Verification items for the finished model (mm, model axes). Round coordinates to 2 decimals unless told otherwise and drop trailing zeros. Write each loop counter-clockwise with the first axis right and the second up, starting at its lowest first coordinate (ties: lowest second). Pieces come first, ordered by that corner, then holes. Notation, with made-up numbers: M 3.25,5 L 11.25,5 A29 cw 11.25,28 Z; hole C -16.5,73 d10. An arc over 180 degrees is marked long. One line per item, written item: value. Start each with the question number.
Item 1: Section check A-A, the plane z = 0.95. State how many separate pieces and enclosed holes the cut face has, then the cut area to 3 significant figures.
Item 2: Thickness scan on probe 1 along X at (y, z) = (254, 1.2); probe 2 along Y at (x, z) = (228.6, 2.45); probe 3 along X at (y, z) = (368.3, 0.7). Record the ranges inside material, lowest first. Write a range as from..to.
Item 3: Gauge pin test, flat ends, axial feed: pin 1 (11.5 mm diameter, centred on x = 571.5, y = 25.4, fed in from +Z) (3 decimals); pin 2 (1 mm diameter, centred on x = 46.5, z = 1, fed in from +Y); pin 3 (6.5 mm diameter, centred on x = 774.7, y = 254, fed in from +Z). Record the tip position at first contact, or that the pin passes through.
Item 4: Section check B-B, the plane x = 585.5. Record the cut outline in (y, z) (3 decimals), then the cut area to 3 significant figures.
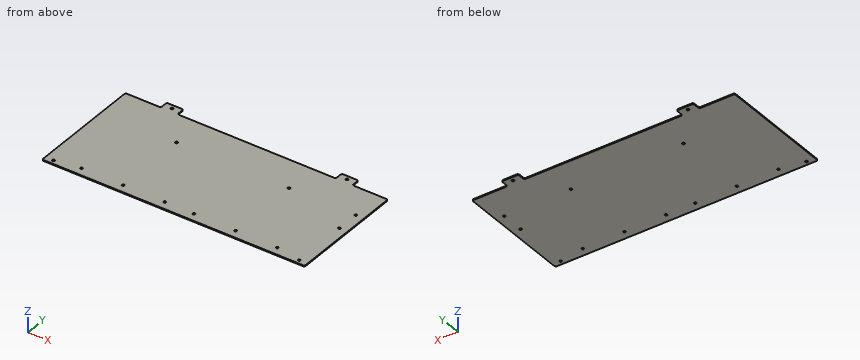
from build123d import *

# Parameters (mm, degrees)
F0_W     = 107.95
F0_H     = 355.6
F0_W_2   = 50.8
F0_H_2   = 25.4
F1_DEPTH = 3.175
F2_D     = 7.1374
F3_R     = 5.08
F5_D     = 7.1374


# Not quite as in the source:
# - a feature names something its author has since deleted; it is built from what else it names


with BuildPart() as f1:
    # F0 (on Top) → F1 (new body)
    with BuildSketch(Plane.XY):
        with Locations((53.975, 177.8)):
            Rectangle(F0_W, F0_H)
        Polygon((107.95, 355.6), (107.95, 0), (400.05, 0), (400.05, 355.6), (158.75, 355.6), align=None)
        with Locations((133.35, 368.3)):
            Rectangle(F0_W_2, F0_H_2)
        Polygon((400.05, 355.6), (400.05, 0), (692.15, 0), (692.15, 355.6), (641.35, 355.6), align=None)
        with Locations((746.125, 177.8)):
            Rectangle(F0_W, F0_H)
        with Locations((666.75, 368.3)):
            Rectangle(F0_W_2, F0_H_2)
    extrude(amount=F1_DEPTH)

    # F2 (through all)
    with Locations(Plane(origin=(0, 0, 0), x_dir=(1, 0, 0), z_dir=(0, 0, -1))):
        with Locations((133.35, -368.3), (666.75, -368.3), (25.4, -12.7), (774.7, -12.7)):
            Hole(F2_D / 2)

    # F3
    f3_edges = [f1.edges().sort_by_distance(p)[0] for p in [
        (0, 355.6, 1.5875),
        (107.95, 355.6, 1.5875),
        (107.95, 381, 1.5875),
        (158.75, 381, 1.5875),
        (158.75, 355.6, 1.5875),
        (692.15, 355.6, 1.5875),
        (692.15, 381, 1.5875),
        (641.35, 381, 1.5875),
        (641.35, 355.6, 1.5875),
        (800.1, 355.6, 1.5875),
        (800.1, 0, 1.5875),
        (0, 0, 1.5875),
    ]]
    fillet(f3_edges, radius=F3_R)

    # F5 (through all)
    with Locations(Plane.XY.offset(3.175)):
        with Locations((571.5, 254), (774.7, 254), (444.5, 25.4), (571.5, 25.4), (698.5, 25.4), (774.7, 184.15), (101.6, 25.4), (228.6, 25.4), (355.6, 25.4), (228.6, 254)):
            Hole(F5_D / 2)


solid = f1.part
Response values:
1. separate pieces: 1
1. enclosed holes: 14
1. area: 287,000 mm2
2. probe 1: x = 0..225.03, 232.17..567.93, 575.07..771.13, 778.27..800.1
2. probe 2: y = 0..21.83, 28.97..250.43, 257.57..355.6
2. probe 3: x = 107.95..129.78, 136.92..158.75, 641.35..663.18, 670.32..692.15
3. pin 1: stops at z = 3.175
3. pin 2: stops at y = 355.6
3. pin 3: passes through
4. outline: M 0,0 L 355.6,0 L 355.6,3.175 L 0,3.175 Z
4. area: 1,130 mm2
